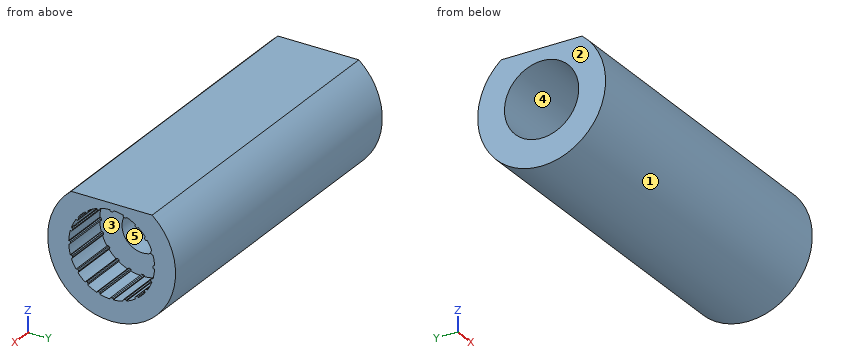
from build123d import *

# Parameters (mm, degrees)
CROQUIS1_R              = 2.25
CROQUIS1_R_2            = 1.25
SALIENTE_EXTRUIR1_DEPTH = 20
CORTAR_EXTRUIR2_DEPTH   = 3
CROQUIS1_3_R            = 2.25
CROQUIS1_3_R_2          = 1.25
CORTAR_EXTRUIR1_DEPTH   = 15.5
CROQUIS1_5_R            = 1.25
CORTAR_EXTRUIR4_DEPTH   = 17


with BuildPart() as part:
    # Croquis1 → Saliente-Extruir1 (new body)
    with BuildSketch(Plane.YZ):
        with BuildLine():
            Line((2.452677109, 3), (-2.452677109, 3))
            ThreePointArc((-2.452677109, 3), (0, -3.875), (2.452677109, 3))
        make_face()
        Circle(CROQUIS1_R, mode=Mode.SUBTRACT)
        Circle(CROQUIS1_R)
        Circle(CROQUIS1_R_2, mode=Mode.SUBTRACT)
        Circle(CROQUIS1_R_2)
    extrude(amount=SALIENTE_EXTRUIR1_DEPTH)

    # Croquis2 → Cortar-Extruir2 (cut)
    with BuildSketch(Plane.YZ.offset(20)):
        with BuildLine():
            Line((-2.498076211, 0.05), (-2.498076211, 0))
            Line((-2.498076211, 0), (-2.498076211, -0.05))
            Line((-2.498076211, -0.05), (-2.548076211, -0.1))
            Line((-2.548076211, -0.1), (-2.598076211, -0.1))
            ThreePointArc((-2.598076211, -0.1), (-2.567989686, -0.406729609), (-2.50181901, -0.70774405))
            Line((-2.50181901, -0.70774405), (-2.454266184, -0.692293201))
            Line((-2.454266184, -0.692293201), (-2.391262509, -0.724395177))
            Line((-2.391262509, -0.724395177), (-2.375811659, -0.771948003))
            Line((-2.375811659, -0.771948003), (-2.360360809, -0.819500828))
            Line((-2.360360809, -0.819500828), (-2.392462785, -0.882504504))
            Line((-2.392462785, -0.882504504), (-2.440015611, -0.897955354))
            ThreePointArc((-2.440015611, -0.897955354), (-2.316616963, -1.180375299), (-2.160666333, -1.446209182))
            Line((-2.160666333, -1.446209182), (-2.120215483, -1.416819919))
            Line((-2.120215483, -1.416819919), (-2.050375371, -1.427881506))
            Line((-2.050375371, -1.427881506), (-2.020986108, -1.468332356))
            Line((-2.020986108, -1.468332356), (-1.991596846, -1.508783206))
            Line((-1.991596846, -1.508783206), (-2.002658433, -1.578623318))
            Line((-2.002658433, -1.578623318), (-2.043109282, -1.608012581))
            ThreePointArc((-2.043109282, -1.608012581), (-1.838477631, -1.838477631), (-1.608012581, -2.043109282))
            Line((-1.608012581, -2.043109282), (-1.578623318, -2.002658433))
            Line((-1.578623318, -2.002658433), (-1.508783206, -1.991596846))
            Line((-1.508783206, -1.991596846), (-1.468332356, -2.020986108))
            Line((-1.468332356, -2.020986108), (-1.427881506, -2.050375371))
            Line((-1.427881506, -2.050375371), (-1.416819919, -2.120215483))
            Line((-1.416819919, -2.120215483), (-1.446209182, -2.160666333))
            ThreePointArc((-1.446209182, -2.160666333), (-1.180375299, -2.316616963), (-0.897955354, -2.440015611))
            Line((-0.897955354, -2.440015611), (-0.882504504, -2.392462785))
            Line((-0.882504504, -2.392462785), (-0.819500828, -2.360360809))
            Line((-0.819500828, -2.360360809), (-0.771948003, -2.375811659))
            Line((-0.771948003, -2.375811659), (-0.724395177, -2.391262509))
            Line((-0.724395177, -2.391262509), (-0.692293201, -2.454266184))
            Line((-0.692293201, -2.454266184), (-0.70774405, -2.50181901))
            ThreePointArc((-0.70774405, -2.50181901), (-0.406729609, -2.567989686), (-0.1, -2.598076211))
            Line((-0.1, -2.598076211), (-0.1, -2.548076211))
            Line((-0.1, -2.548076211), (-0.05, -2.498076211))
            Line((-0.05, -2.498076211), (0, -2.498076211))
            Line((0, -2.498076211), (0.05, -2.498076211))
            Line((0.05, -2.498076211), (0.1, -2.548076211))
            Line((0.1, -2.548076211), (0.1, -2.598076211))
            ThreePointArc((0.1, -2.598076211), (0.406729609, -2.567989686), (0.70774405, -2.50181901))
            Line((0.70774405, -2.50181901), (0.692293201, -2.454266184))
            Line((0.692293201, -2.454266184), (0.724395177, -2.391262509))
            Line((0.724395177, -2.391262509), (0.771948003, -2.375811659))
            Line((0.771948003, -2.375811659), (0.819500828, -2.360360809))
            Line((0.819500828, -2.360360809), (0.882504504, -2.392462785))
            Line((0.882504504, -2.392462785), (0.897955354, -2.440015611))
            ThreePointArc((0.897955354, -2.440015611), (1.180375299, -2.316616963), (1.446209182, -2.160666333))
            Line((1.446209182, -2.160666333), (1.416819919, -2.120215483))
            Line((1.416819919, -2.120215483), (1.427881506, -2.050375371))
            Line((1.427881506, -2.050375371), (1.468332356, -2.020986108))
            Line((1.468332356, -2.020986108), (1.508783206, -1.991596846))
            Line((1.508783206, -1.991596846), (1.578623318, -2.002658433))
            Line((1.578623318, -2.002658433), (1.608012581, -2.043109282))
            ThreePointArc((1.608012581, -2.043109282), (1.838477631, -1.838477631), (2.043109282, -1.608012581))
            Line((2.043109282, -1.608012581), (2.002658433, -1.578623318))
            Line((2.002658433, -1.578623318), (1.991596846, -1.508783206))
            Line((1.991596846, -1.508783206), (2.020986108, -1.468332356))
            Line((2.020986108, -1.468332356), (2.050375371, -1.427881506))
            Line((2.050375371, -1.427881506), (2.120215483, -1.416819919))
            Line((2.120215483, -1.416819919), (2.160666333, -1.446209182))
            ThreePointArc((2.160666333, -1.446209182), (2.316616963, -1.180375299), (2.440015611, -0.897955354))
            Line((2.440015611, -0.897955354), (2.392462785, -0.882504504))
            Line((2.392462785, -0.882504504), (2.360360809, -0.819500828))
            Line((2.360360809, -0.819500828), (2.375811659, -0.771948003))
            Line((2.375811659, -0.771948003), (2.391262509, -0.724395177))
            Line((2.391262509, -0.724395177), (2.454266184, -0.692293201))
            Line((2.454266184, -0.692293201), (2.50181901, -0.70774405))
            ThreePointArc((2.50181901, -0.70774405), (2.567989686, -0.406729609), (2.598076211, -0.1))
            Line((2.598076211, -0.1), (2.548076211, -0.1))
            Line((2.548076211, -0.1), (2.498076211, -0.05))
            Line((2.498076211, -0.05), (2.498076211, 0))
            Line((2.498076211, 0), (2.498076211, 0.05))
            Line((2.498076211, 0.05), (2.548076211, 0.1))
            Line((2.548076211, 0.1), (2.598076211, 0.1))
            ThreePointArc((2.598076211, 0.1), (2.567989686, 0.406729609), (2.50181901, 0.70774405))
            Line((2.50181901, 0.70774405), (2.454266184, 0.692293201))
            Line((2.454266184, 0.692293201), (2.391262509, 0.724395177))
            Line((2.391262509, 0.724395177), (2.375811659, 0.771948003))
            Line((2.375811659, 0.771948003), (2.360360809, 0.819500828))
            Line((2.360360809, 0.819500828), (2.392462785, 0.882504504))
            Line((2.392462785, 0.882504504), (2.440015611, 0.897955354))
            ThreePointArc((2.440015611, 0.897955354), (2.316616963, 1.180375299), (2.160666333, 1.446209182))
            Line((2.160666333, 1.446209182), (2.120215483, 1.416819919))
            Line((2.120215483, 1.416819919), (2.050375371, 1.427881506))
            Line((2.050375371, 1.427881506), (2.020986108, 1.468332356))
            Line((2.020986108, 1.468332356), (1.991596846, 1.508783206))
            Line((1.991596846, 1.508783206), (2.002658433, 1.578623318))
            Line((2.002658433, 1.578623318), (2.043109282, 1.608012581))
            ThreePointArc((2.043109282, 1.608012581), (1.838477631, 1.838477631), (1.608012581, 2.043109282))
            Line((1.608012581, 2.043109282), (1.578623318, 2.002658433))
            Line((1.578623318, 2.002658433), (1.508783206, 1.991596846))
            Line((1.508783206, 1.991596846), (1.468332356, 2.020986108))
            Line((1.468332356, 2.020986108), (1.427881506, 2.050375371))
            Line((1.427881506, 2.050375371), (1.416819919, 2.120215483))
            Line((1.416819919, 2.120215483), (1.446209182, 2.160666333))
            ThreePointArc((1.446209182, 2.160666333), (1.180375299, 2.316616963), (0.897955354, 2.440015611))
            Line((0.897955354, 2.440015611), (0.882504504, 2.392462785))
            Line((0.882504504, 2.392462785), (0.819500828, 2.360360809))
            Line((0.819500828, 2.360360809), (0.771948003, 2.375811659))
            Line((0.771948003, 2.375811659), (0.724395177, 2.391262509))
            Line((0.724395177, 2.391262509), (0.692293201, 2.454266184))
            Line((0.692293201, 2.454266184), (0.70774405, 2.50181901))
            ThreePointArc((0.70774405, 2.50181901), (0.406729609, 2.567989686), (0.1, 2.598076211))
            Line((0.1, 2.598076211), (0.1, 2.548076211))
            Line((0.1, 2.548076211), (0.05, 2.498076211))
            Line((0.05, 2.498076211), (0, 2.498076211))
            Line((0, 2.498076211), (-0.05, 2.498076211))
            Line((-0.05, 2.498076211), (-0.1, 2.548076211))
            Line((-0.1, 2.548076211), (-0.1, 2.598076211))
            ThreePointArc((-0.1, 2.598076211), (-0.406729609, 2.567989686), (-0.70774405, 2.50181901))
            Line((-0.70774405, 2.50181901), (-0.692293201, 2.454266184))
            Line((-0.692293201, 2.454266184), (-0.724395177, 2.391262509))
            Line((-0.724395177, 2.391262509), (-0.771948003, 2.375811659))
            Line((-0.771948003, 2.375811659), (-0.819500828, 2.360360809))
            Line((-0.819500828, 2.360360809), (-0.882504504, 2.392462785))
            Line((-0.882504504, 2.392462785), (-0.897955354, 2.440015611))
            ThreePointArc((-0.897955354, 2.440015611), (-1.180375299, 2.316616963), (-1.446209182, 2.160666333))
            Line((-1.446209182, 2.160666333), (-1.416819919, 2.120215483))
            Line((-1.416819919, 2.120215483), (-1.427881506, 2.050375371))
            Line((-1.427881506, 2.050375371), (-1.468332356, 2.020986108))
            Line((-1.468332356, 2.020986108), (-1.508783206, 1.991596846))
            Line((-1.508783206, 1.991596846), (-1.578623318, 2.002658433))
            Line((-1.578623318, 2.002658433), (-1.608012581, 2.043109282))
            ThreePointArc((-1.608012581, 2.043109282), (-1.838477631, 1.838477631), (-2.043109282, 1.608012581))
            Line((-2.043109282, 1.608012581), (-2.002658433, 1.578623318))
            Line((-2.002658433, 1.578623318), (-1.991596846, 1.508783206))
            Line((-1.991596846, 1.508783206), (-2.020986108, 1.468332356))
            Line((-2.020986108, 1.468332356), (-2.050375371, 1.427881506))
            Line((-2.050375371, 1.427881506), (-2.120215483, 1.416819919))
            Line((-2.120215483, 1.416819919), (-2.160666333, 1.446209182))
            ThreePointArc((-2.160666333, 1.446209182), (-2.316616963, 1.180375299), (-2.440015611, 0.897955354))
            Line((-2.440015611, 0.897955354), (-2.392462785, 0.882504504))
            Line((-2.392462785, 0.882504504), (-2.360360809, 0.819500828))
            Line((-2.360360809, 0.819500828), (-2.375811659, 0.771948003))
            Line((-2.375811659, 0.771948003), (-2.391262509, 0.724395177))
            Line((-2.391262509, 0.724395177), (-2.454266184, 0.692293201))
            Line((-2.454266184, 0.692293201), (-2.50181901, 0.70774405))
            ThreePointArc((-2.50181901, 0.70774405), (-2.567989686, 0.406729609), (-2.598076211, 0.1))
            Line((-2.598076211, 0.1), (-2.548076211, 0.1))
            Line((-2.548076211, 0.1), (-2.498076211, 0.05))
        make_face()
    extrude(amount=-CORTAR_EXTRUIR2_DEPTH, mode=Mode.SUBTRACT)

    # Croquis1<3> → Cortar-Extruir1 (cut)
    with BuildSketch(Plane.YZ):
        with Locations(Location((0, 0, 0), (0, 0, 90))):
            Circle(CROQUIS1_3_R)
        with Locations(Location((0, 0, 0), (0, 0, 90))):
            Circle(CROQUIS1_3_R_2, mode=Mode.SUBTRACT)
    extrude(amount=CORTAR_EXTRUIR1_DEPTH, mode=Mode.SUBTRACT)

    # Croquis1<5> → Cortar-Extruir4 (cut)
    with BuildSketch(Plane.YZ):
        with Locations(Location((0, 0, 0), (0, 0, 270))):
            Circle(CROQUIS1_5_R)
    extrude(amount=CORTAR_EXTRUIR4_DEPTH, mode=Mode.SUBTRACT)


solid = part.part
Design review of the part built by this model. Coordinates are the model's own, in mm. Face numbers are marked on the shaded views. A direction names the side the tool comes from. Round coordinates to 2 decimals unless told otherwise and drop trailing zeros. Loops run counter-clockwise (first coordinate to the right, second up) from the corner with the lowest first, then second, coordinate; pieces in that order, holes last. Notation, with made-up numbers: (-38.75, 63.25) - (-19.75, 63.25) arc R19 ccw to (-19.75, 82.25) - close; hole circle Ø8 at (11, 45). An arc over 180 degrees is marked (long way). One line per item, written item: value. Start each with the question number.
1) To check wall thickness, follow L1, parallel to Y at x = 8, z = 0 (3 decimals); L2, parallel to Y at x = 16.55, z = 0 (3 decimals); L3, parallel to Z at x = 9, y = 0.25. State the ranges of each line that lie inside material, in increasing order. Write a range as from..to.
2) Consider section A-A on y = -0.5. Give the boundary of the cut face in (x, z), then the cut area to 3 significant figures.
3) Draft analysis for pull direction Y (two halves, no side actions). For the marked faces 1, 2 and 3, state which applies: +Y half, -Y half, draft (parallel to the pull), parting line (faces both ways), or undercut.
4) Consider section B-B on x = 6. Give the boundary of the cut face in (y, z) (3 decimals), then the cut area to 3 significant figures.
5) For the marked faces 4 and 5, list the 3-axis set-ups (+Z, -Z, +X, -X, +Y, -Y) from which the entire face can be reached by the end or side of a thin tool; tool diameter is ignored.
6) Insertion check: pin 1 Ø1.5 at (y, z) = (-1, -0.5) entering from +X; pin 2 Ø2 at (x, z) = (17.5, 1.5) entering from -Y; pin 3 Ø2 at (x, z) = (2.5, 2) entering from +Y. Each pin has a flat end and moves straight along its axis. Give the tip position at first contact, or say it passes through.
Reported:
1. L1: y = -3.875..-2.25, 2.25..3.875
1. L2: y = -3.875..-1.25, 1.25..3.875
1. L3: z = -3.87..-2.24, 2.24..3
2. outline: (0, -3.84) - (20, -3.84) - (20, -2.55) - (17, -2.55) - (17, -1.15) - (15.5, -1.15) - (15.5, -2.19) - (0, -2.19) - close; (0, 2.19) - (15.5, 2.19) - (15.5, 1.15) - (17, 1.15) - (17, 2.55) - (20, 2.55) - (20, 3) - (0, 3) - close
2. area: 50.1 mm^2
3. face 1: parting line
3. face 2: draft
3. face 3: undercut
4. outline: (-2.453, 3) arc R3.875 ccw (long way) to (2.453, 3) - close; hole circle Ø4.5 at (0, 0)
4. area: 28.3 mm^2
5. face 4: -X
5. face 5: +X, -X
6. pin 1: stops at x = 17
6. pin 2: stops at y = -3.84
6. pin 3: stops at y = 3.74
